from build123d import *

# Parameters (mm, degrees)
SKETCH1_R           = 21
BOSS_EXTRUDE1_DEPTH = 40
BOSS_EXTRUDE2_DEPTH = 2
SKETCH3_R           = 4
BOSS_EXTRUDE3_DEPTH = 20
SKETCH4_R           = 2
CUT_EXTRUDE1_DEPTH  = 10
SKETCH5_R           = 21.25
BOSS_EXTRUDE4_DEPTH = 75
SKETCH6_R           = 22.5
SKETCH6_R_2         = 21.25
BOSS_EXTRUDE5_DEPTH = 34


with BuildPart() as part:
    # Sketch1 → Boss-Extrude1 (new body)
    with BuildSketch(Plane(origin=(0, 0, 0), x_dir=(0, 0, -1), z_dir=(1, 0, 0))):
        Circle(SKETCH1_R)
    extrude(amount=BOSS_EXTRUDE1_DEPTH)

    # Sketch2 → Boss-Extrude2 (add)
    with BuildSketch(Plane(origin=(40, 0, 0), x_dir=(0, 0, -1), z_dir=(1, 0, 0))):
        with BuildLine():
            Line((-11.5, 4.898979486), (-11.5, -4.898979486))
            ThreePointArc((-11.5, -4.898979486), (0, -12.5), (11.5, -4.898979486))
            Line((11.5, -4.898979486), (11.5, 4.898979486))
            ThreePointArc((11.5, 4.898979486), (0, 12.5), (-11.5, 4.898979486))
        make_face()
    extrude(amount=BOSS_EXTRUDE2_DEPTH)

    # Sketch3 → Boss-Extrude3 (add)
    with BuildSketch(Plane(origin=(42, 0, 0), x_dir=(0, 0, -1), z_dir=(1, 0, 0))):
        Circle(SKETCH3_R)
    extrude(amount=BOSS_EXTRUDE3_DEPTH)

    # Sketch4 → Cut-Extrude1 (cut)
    with BuildSketch(Plane(origin=(40, 0, 0), x_dir=(0, 0, -1), z_dir=(1, 0, 0))):
        with Locations((-12.374368671, 12.374368671)):
            Circle(SKETCH4_R)
        with Locations((12.374368671, 12.374368671)):
            Circle(SKETCH4_R)
        with Locations((12.374368671, -12.374368671)):
            Circle(SKETCH4_R)
        with Locations((-12.374368671, -12.374368671)):
            Circle(SKETCH4_R)
    extrude(amount=-CUT_EXTRUDE1_DEPTH, mode=Mode.SUBTRACT)

    # Sketch5 → Boss-Extrude4 (add)
    with BuildSketch(Plane.ZY):
        Circle(SKETCH5_R)
    extrude(amount=BOSS_EXTRUDE4_DEPTH)

    # Sketch6 → Boss-Extrude5 (add)
    with BuildSketch(Plane(origin=(-7, 0, 0), x_dir=(0, 0, -1), z_dir=(1, 0, 0))):
        Circle(SKETCH6_R)
        Circle(SKETCH6_R_2, mode=Mode.SUBTRACT)
    extrude(amount=-BOSS_EXTRUDE5_DEPTH)


solid = part.part
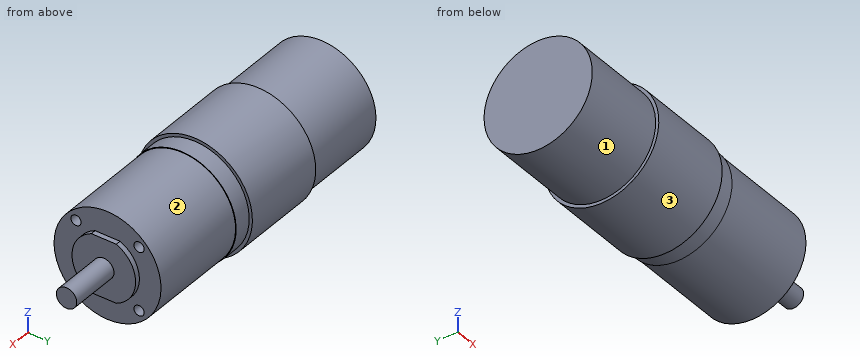
The listing builds one solid part. Answer for the finished solid, in the listing's coordinates (mm). Face numbers are marked on the shaded views. A direction names the side the tool comes from. Coordinates: 2 decimals unless noted, no trailing zeros. Loops run counter-clockwise (first coordinate to the right, second up) from the corner with the lowest first, then second, coordinate; pieces in that order, holes last. Notation, with made-up numbers: M -5,9 L 51,9 A27 cw 51,35 Z; hole C 47.5,42 d9. An arc over 180 degrees is marked long. Answer in a Markdown table with one row per item.
1) Find the intervals of material crossed by probe 1 along X at (y, z) = (3.5, 16.5); probe 2 along X at (y, z) = (11, -0.5); probe 3 along Y at (x, z) = (12, 0), in increasing order.
Answers below:
| item | result |
|---|---|
| probe 1 | -75 to 40 |
| probe 2 | -75 to 42 |
| probe 3 | -21 to 21 |
2) Find section A-A (y = 0). Determine the outline of the cut face in (x, z).
Answers below:
| item | result |
|---|---|
| outline | M -75,-21.25 L -41,-21.25 L -41,-22.5 L -7,-22.5 L -7,-21.25 L 0,-21.25 L 0,-21 L 40,-21 L 40,-11.5 L 42,-11.5 L 42,-4 L 62,-4 L 62,4 L 42,4 L 42,11.5 L 40,11.5 L 40,21 L 0,21 L 0,21.25 L -7,21.25 L -7,22.5 L -41,22.5 L -41,21.25 L -75,21.25 Z |
3) Find section B-B (z = 0). Determine the outline of the cut face in (x, y), then the cut area to 3 significant figures.
Answers below:
| item | result |
|---|---|
| outline | M -75,-21.25 L -41,-21.25 L -41,-22.5 L -7,-22.5 L -7,-21.25 L 0,-21.25 L 0,-21 L 40,-21 L 40,-12.5 L 42,-12.5 L 42,-4 L 62,-4 L 62,4 L 42,4 L 42,12.5 L 40,12.5 L 40,21 L 0,21 L 0,21.25 L -7,21.25 L -7,22.5 L -41,22.5 L -41,21.25 L -75,21.25 Z |
| area | 5,160 mm^2 |
4) Find section D-D (z = -6.5). Determine the outline of the cut face in (x, y), then the cut area to 3 significant figures.
Answers below:
| item | result |
|---|---|
| outline | M -75,-20.23 L -41,-20.23 L -41,-21.54 L -7,-21.54 L -7,-20.23 L 0,-20.23 L 0,-19.97 L 40,-19.97 L 40,-10.68 L 42,-10.68 L 42,10.68 L 40,10.68 L 40,19.97 L 0,19.97 L 0,20.23 L -7,20.23 L -7,21.54 L -41,21.54 L -41,20.23 L -75,20.23 Z |
| area | 4,760 mm^2 |
5) Which of the six approach directions +Z, -Z, +X, -X, +Y, -Y give full straight-line access (tool end or side, diameter ignored) to the marked faces 1, 2 and 3?
Answers below:
| item | result |
|---|---|
| face 1 | -X |
| face 2 | +X |
| face 3 | +X, -X |
6) Given pin 1 (1.5 mm diameter, centred on x = -38, z = 1, fed in from -Y); pin 2 (5 mm diameter, centred on y = -12.37, z = -12.37, fed in from +X); pin 3 (7 mm diameter, centred on y = -6, z = -5, fed in from +X), each flat-ended and moving along its own axis, determine where each tip first touches the part or whether it passes through.
Answers below:
| item | result |
|---|---|
| pin 1 | y = -22.5 |
| pin 2 | x = 40 |
| pin 3 | x = 42 |
7) Find section C-C (x = -4). Determine the outline of the cut face in (y, z).
Answers below:
| item | result |
|---|---|
| outline | C 0,0 d42.5 |
